```python
from build123d import *

# Parameters (mm, degrees)
CROQUIS3_R                 = 27.75
CROQUIS3_R_2               = 25
SALIENTE_EXTRUIR1_DEPTH    = 15
CROQUIS4_R                 = 33
CROQUIS4_R_2               = 25
SALIENTE_EXTRUIR2_DEPTH    = 5
CROQUIS5_R                 = 33
CROQUIS5_R_2               = 28
SALIENTE_EXTRUIR3_DEPTH    = 53
CROQUIS6_W                 = 5
CROQUIS6_H                 = 7
CROQUIS6_W_2               = 7
CROQUIS6_H_2               = 5
SALIENTE_EXTRUIR4_DEPTH    = 15
CROQUIS7_R                 = 1.5
CORTAR_EXTRUIR1_DEPTH      = 163.497884602
CROQUIS8_R                 = 1.5
CORTAR_EXTRUIR2_DEPTH      = 163.497884602
CORTAR_EXTRUIR3_DEPTH      = 163.497884602
CORTAR_EXTRUIR3_DEPTH_BACK = 163.497884602
CROQUIS9_R                 = 1.5
CORTAR_EXTRUIR4_DEPTH      = 163.497884691
CORTAR_EXTRUIR4_DEPTH_BACK = 163.497884691
CROQUIS10_R                = 1.5


with BuildPart() as part:
    # Croquis3 → Saliente-Extruir1 (new body)
    with BuildSketch(Plane(origin=(0, 0, 0), x_dir=(1, 0, 0), z_dir=(0, 1, 0))):
        with Locations(Location((0, 0, 0), (0, 0, 270))):
            Circle(CROQUIS3_R)
        with Locations(Location((0, 0, 0), (0, 0, 270))):
            Circle(CROQUIS3_R_2, mode=Mode.SUBTRACT)
    extrude(amount=SALIENTE_EXTRUIR1_DEPTH)

    # Croquis4 → Saliente-Extruir2 (add)
    with BuildSketch(Plane(origin=(0, 15, 0), x_dir=(1, 0, 0), z_dir=(0, 1, 0))):
        with Locations(Location((0, 0, 0), (0, 0, 270))):
            Circle(CROQUIS4_R)
        with Locations(Location((0, 0, 0), (0, 0, 270))):
            Circle(CROQUIS4_R_2, mode=Mode.SUBTRACT)
    extrude(amount=SALIENTE_EXTRUIR2_DEPTH)

    # Croquis5 → Saliente-Extruir3 (add)
    with BuildSketch(Plane(origin=(0, 20, 0), x_dir=(1, 0, 0), z_dir=(0, 1, 0))):
        with Locations(Location((0, 0, 0), (0, 0, 270))):
            Circle(CROQUIS5_R)
        with Locations(Location((0, 0, 0), (0, 0, 270))):
            Circle(CROQUIS5_R_2, mode=Mode.SUBTRACT)
    extrude(amount=SALIENTE_EXTRUIR3_DEPTH)

    # Croquis6 → Saliente-Extruir4 (add)
    with BuildSketch(Plane.XZ.offset(-15)):
        with Locations((27.75, 0)):
            Rectangle(CROQUIS6_W, CROQUIS6_H)
        with Locations((0, 27.75)):
            Rectangle(CROQUIS6_W_2, CROQUIS6_H_2)
        with Locations((0, -27.75)):
            Rectangle(CROQUIS6_W_2, CROQUIS6_H_2)
        with Locations((-27.75, 0)):
            Rectangle(CROQUIS6_W, CROQUIS6_H)
    extrude(amount=SALIENTE_EXTRUIR4_DEPTH)

    # Simetría2: part across plane


with BuildPart() as part_1:
    add(part.part)
    add(part.part.mirror(Plane.ZX.offset(73)))

    # Croquis7 → Cortar-Extruir1 (cut, through all)
    with BuildSketch(Plane.ZY.offset(30.25)):
        with Locations((0, 7.5)):
            Circle(CROQUIS7_R)
    extrude(amount=-CORTAR_EXTRUIR1_DEPTH, mode=Mode.SUBTRACT)

    # Croquis8 → Cortar-Extruir2 (cut, through all)
    with BuildSketch(Plane(origin=(0, 0, -30.25), x_dir=(-1, 0, 0), z_dir=(0, 0, -1))):
        with Locations((0, 7.5)):
            Circle(CROQUIS8_R)
    extrude(amount=-CORTAR_EXTRUIR2_DEPTH, mode=Mode.SUBTRACT)

    # Croquis9 → Cortar-Extruir3 (cut, two sides: drawn at the far end of the back side and taken through both)
    with BuildSketch(Plane.ZY.offset(30.25).offset(-CORTAR_EXTRUIR3_DEPTH_BACK)):
        with Locations((0, 138.5)):
            Circle(CROQUIS9_R)
    extrude(amount=CORTAR_EXTRUIR3_DEPTH + CORTAR_EXTRUIR3_DEPTH_BACK, mode=Mode.SUBTRACT)

    # Croquis10 → Cortar-Extruir4 (cut, two sides: drawn at the far end of the back side and taken through both)
    with BuildSketch(Plane.XY.offset(30.25).offset(-CORTAR_EXTRUIR4_DEPTH_BACK)):
        with Locations((0, 138.5)):
            Circle(CROQUIS10_R)
    extrude(amount=CORTAR_EXTRUIR4_DEPTH + CORTAR_EXTRUIR4_DEPTH_BACK, mode=Mode.SUBTRACT)


solid = part_1.part
```
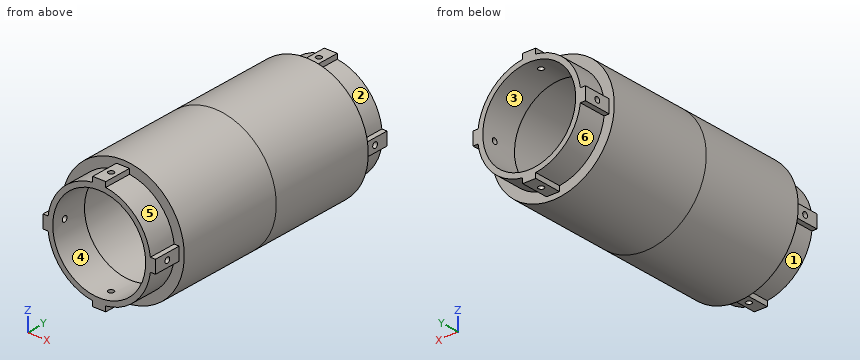
Input: part model. Units: mm. Frame: model coordinates. Face numbers are marked on the shaded views. A direction names the side the tool comes from. Give positions to 0.01 mm unless a question says otherwise; leave off trailing zeros. Order: outer loops, then holes, each group sorted by start corner. A loop starts at its lowest first (then second) coordinate and runs counter-clockwise, first axis right, second up. Notation, with made-up numbers: (9, 56) -> (50, 56) arc R23 cw to (50, 65) -> close; hole circle Ø1 at (68.5, 11). An arc over 180 degrees is marked (long way). Write each question's results on one line, items separated by ' | '. Start each with the question number.
Item 1: Cut plane D-D on y = 53. Return the cut outline in (x, z), then the cut area to 3 significant figures.
Item 2: Mould query, pull axis X, two halves, no side actions, for the marked faces 3, 4, 5 and 6. Classes: pulls with the +X half, pulls with the -X half, needs draft (parallel to the pull), parting line crosses it, or undercut.
Item 3: Line query: line 1 (Y direction, x = 26.8, z = 0); line 2 (Y direction, x = 20.5, z = 18); line 3 (X direction, y = 135.25, z = 0). Output: solid intervals per line, ascending.
Item 4: Cut plane A-A on y = 7.5. Give the number of separate pieces and of enclosed holes in the cut face, then the cut area to 3 significant figures.
Item 5: Contact query for flat-ended pins moving along their axis: P1, Ø5.5, axis at x = -1, y = 138.5, coming from the +Z side; P2, Ø1, axis at x = -12, y = 72.5, coming from the +Z side; P3, Ø1.5, axis at y = 93.5, z = 23, coming from the -X side. Output: stop coordinate, or through.
Item 6: Set-up query: the marked faces 1 and 2. Return all of +Z, -Z, +X, -X, +Y, -Y with unobstructed straight access to the full face (end or side cutting, diameter ignored); none if empty.
Item 7: Cut plane B-B on z = 6. Return the cut outline in (x, y), then the cut area to 3 significant figures.
Established:
1) outline: circle Ø66 at (0, 0); hole circle Ø56 at (0, 0) | area: 958 mm^2
2) face 3: undercut | face 4: undercut | face 5: pulls with the +X half | face 6: pulls with the -X half
3) line 1: 0 to 6, 9 to 20, 126 to 137, 140 to 146 | line 2: 0 to 20, 126 to 146 | line 3: -30.25 to -25, 25 to 30.25
4) separate pieces: 4 | enclosed holes: 0 | area: 465 mm^2
5) P1: z = 30.25 | P2: z = 30.93 | P3: x = -24.37
6) face 1: -Z, -X, -Y | face 2: +Z, +X, +Y
7) outline: (-32.45, 15) -> (-27.09, 15) -> (-27.09, 0) -> (-24.27, 0) -> (-24.27, 20) -> (-27.35, 20) -> (-27.35, 126) -> (-24.27, 126) -> (-24.27, 146) -> (-27.09, 146) -> (-27.09, 131) -> (-32.45, 131) -> close; (24.27, 0) -> (27.09, 0) -> (27.09, 15) -> (32.45, 15) -> (32.45, 131) -> (27.09, 131) -> (27.09, 146) -> (24.27, 146) -> (24.27, 126) -> (27.35, 126) -> (27.35, 20) -> (24.27, 20) -> close | area: 1,410 mm^2
